Can you work these out from the model? Positions are in its coordinate system, mm. A direction names the side the tool comes from. Give positions to 0.01 mm unless a question says otherwise; leave off trailing zeros. Loops run counter-clockwise (first coordinate to the right, second up) from the corner with the lowest first, then second, coordinate; pieces in that order, holes last. Notation, with made-up numbers: (7.5, -29) -> (19.5, -29) arc R25 cw to (19.5, -15) -> close; hole circle Ø4 at (52, 41). An arc over 180 degrees is marked (long way). Return JSON: item names as keys, results as strings. Group by question number.
Q1. Thinking about a two-plate mould opening in X: for faces 3 (the flat face through (1, 2, 1)), 4 (the flat face through (0, 10, 1)), 5 (the cylindrical face through (-2.44, 9.4, -0.54)), which applies, pulls with the +X half, pulls with the -X half, needs draft (parallel to the pull), parting line crosses it, or undercut?
Q2. Will these pins go through, and if not, where does the flat tip stop? pin 1 (1.4 mm diameter, centred on x = 0, z = 0, fed in from +Y); pin 2 (2 mm diameter, centred on y = 12.5, z = -1.5, fed in from +X); pin 3 (1 mm diameter, centred on y = 15, z = 1, fed in from -X).
Q3. Which directions (+Z, -Z, +X, -X, +Y, -Y) give clear straight access to the entire face, cutting with the end or side of a thin tool? Please do faces 1 (the cylindrical face through (-0.83, 13.55, -0.18)), 2 (the cylindrical face through (-1.22, 5.94, -0.27)).
Q4. Suppose I cut it at A-A, the plane x = 0. Please give me the cut outline in (y, z), and give its area (3 significant figures).
Q5. I need wall thicknesses on line 1 along X through (y, z) = (13, 0); line 2 along X through (y, z) = (2.5, -0.05); line 3 along Y through (x, z) = (-0.65, -0.7). Which ranges of each line are inside material? Lowest first, please. Write a range as [from, to].
Q6. Suppose I cut it at B-B, the plane z = 0. Please give me the cut outline in (x, y).
Q7. Suppose I cut it at C-C, the plane y = 14. Please give me the cut outline in (x, z).
Q8. Suppose I cut it at D-D, the plane z = 1.5. Please give me the cut outline in (x, y), and give its area (3 significant figures).
```python
from build123d import *

# Parameters (mm, degrees)
SKETCH_1_R          = 1.25
EXTRUDE_1_DEPTH     = 2
SKETCH_2_R          = 2.5
EXTRUDE_2_DEPTH     = 15
SKETCH_3_R          = 0.85
CUT_EXTRUDE_1_DEPTH = 8
SKETCH_1_3_R        = 1.25
CUT_EXTRUDE_2_DEPTH = 10


with BuildPart() as part:
    # Sketch 1 → Extrude 1 (new body)
    with BuildSketch(Plane(origin=(0, 0, 0), x_dir=(1, 0, 0), z_dir=(0, 1, 0))):
        with Locations(Location((0, 0, 0), (0, 0, 270))):
            Circle(SKETCH_1_R)
    extrude(amount=EXTRUDE_1_DEPTH)

    # Sketch 2 → Extrude 2 (add)
    with BuildSketch(Plane(origin=(0, 2, 0), x_dir=(1, 0, 0), z_dir=(0, 1, 0))):
        with Locations(Location((0, 0, 0), (0, 0, 270))):
            Circle(SKETCH_2_R)
    extrude(amount=EXTRUDE_2_DEPTH)

    # Sketch 3 → Cut-Extrude 1 (cut)
    with BuildSketch(Plane(origin=(0, 17, 0), x_dir=(1, 0, 0), z_dir=(0, 1, 0))):
        with Locations(Location((0, 0, 0), (0, 0, 270))):
            Circle(SKETCH_3_R)
    extrude(amount=-CUT_EXTRUDE_1_DEPTH, mode=Mode.SUBTRACT)

    # Sketch 1_3 → Cut-Extrude 2 (cut)
    with BuildSketch(Plane(origin=(0, 0, 0), x_dir=(1, 0, 0), z_dir=(0, 1, 0))):
        with Locations(Location((0, 0, 0), (0, 0, 270))):
            Circle(SKETCH_1_3_R)
    extrude(amount=CUT_EXTRUDE_2_DEPTH, mode=Mode.SUBTRACT)


solid = part.part
```
Ans:
{
 "1": {"face 3": "needs draft", "face 4": "undercut", "face 5": "parting line crosses it"},
 "2": {"pin 1": "passes through", "pin 2": "stops at x = 2.45", "pin 3": "stops at x = -2.45"},
 "3": {"face 1": "+Y, -Y", "face 2": "-Y"},
 "4": {"outline": "(2, -2.5) -> (17, -2.5) -> (17, -0.85) -> (10, -0.85) -> (10, -1.25) -> (2, -1.25) -> close; (2, 1.25) -> (10, 1.25) -> (10, 0.85) -> (17, 0.85) -> (17, 2.5) -> (2, 2.5) -> close", "area": "43.1 mm^2"},
 "5": {"line 1": "x = [-2.5, -0.85], [0.85, 2.5]", "line 2": "x = [-2.5, -1.25], [1.25, 2.5]", "line 3": "y = [10, 17]"},
 "6": {"outline": "(-2.5, 2) -> (-1.25, 2) -> (-1.25, 10) -> (-0.85, 10) -> (-0.85, 17) -> (-2.5, 17) -> close; (0.85, 10) -> (1.25, 10) -> (1.25, 2) -> (2.5, 2) -> (2.5, 17) -> (0.85, 17) -> close"},
 "7": {"outline": "circle Ø5 at (0, 0); hole circle Ø1.7 at (0, 0)"},
 "8": {"outline": "(-2, 2) -> (2, 2) -> (2, 17) -> (-2, 17) -> close", "area": "60.0 mm^2"}
}
